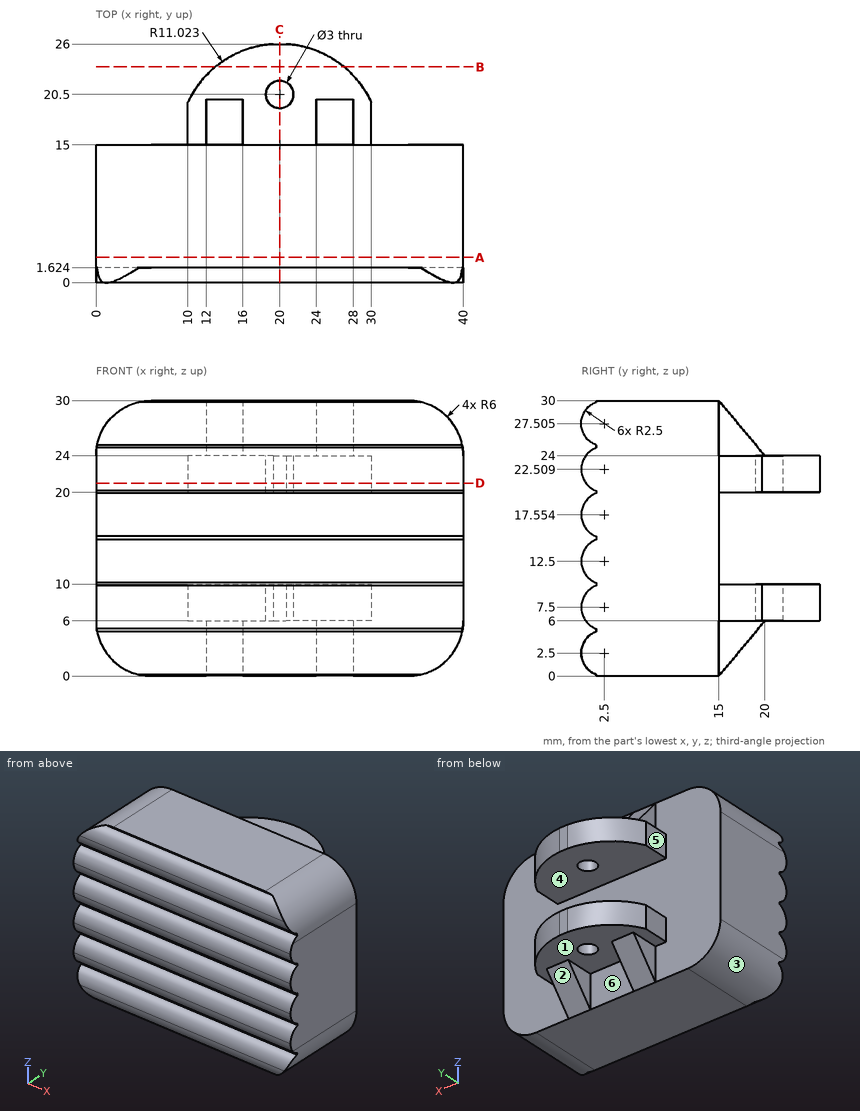
Geometry: see drawing. Coordinates: mm, zero at the bounding-box minimum. A direction names the side the tool comes from. Give positions to 0.01 mm unless a question says otherwise; leave off trailing zeros. Loops run counter-clockwise (first coordinate to the right, second up) from the corner with the lowest first, then second, coordinate; pieces in that order, holes last. Notation, with made-up numbers: (65, 87.25) - (98, 87.25) arc R13 ccw to (98, 94.25) - close; hole circle Ø11 at (-23.5, 16). An arc over 180 degrees is marked (long way). Use CSV: the item, a comma, the result in double quotes.
1) Pin query (flat end, axial travel): P1, Ø1, axis at y = 8.5, z = 27, coming from the +X side (1 decimal); P2, Ø8, axis at y = 22, z = 19, coming from the -X side; P3, Ø4, axis at y = 16.5, z = 1.5, coming from the +X side. Return the tip coordinate at first contact, or that it passes through.
Worked out:
P1,"stops at x = 39.5"
P2,"stops at x = 10"
P3,"stops at x = 39.09"
2) Line query: line 1 (Y direction, x = 20, z = 8); line 2 (Z direction, x = 23.5, y = 21.75); line 3 (X direction, y = 16.75, z = 8.5). Output: solid intervals per line, ascending.
Worked out:
line 1,"y = 0.05 to 19, 22 to 26"
line 2,"z = 6 to 10, 20 to 24"
line 3,"x = 10 to 30"
3) Cut plane C-C (x = 20). Count the separate pieces of the cut face and the enclosed holes in it.
Worked out:
separate pieces,"3"
enclosed holes,"0"
4) Cut plane A-A (y = 2.75). Output: boundary loops of the cut face in (x, z), and give its area (3 significant figures).
Worked out:
outline,"(0, 6) arc R6 ccw to (6, 0) - (34, 0) arc R6 ccw to (40, 6) - (40, 24) arc R6 ccw to (34, 30) - (6, 30) arc R6 ccw to (0, 24) - close"
area,"1,170 mm^2"
5) Cut plane B-B (y = 23.5). Output: boundary loops of the cut face in (x, z), and give its area (3 significant figures).
Worked out:
outline,"(12.98, 6) - (27.02, 6) - (27.02, 10) - (12.98, 10) - close; (12.98, 20) - (27.02, 20) - (27.02, 24) - (12.98, 24) - close"
area,"112 mm^2"
6) Set-up query: the marked faces 4, 5 and 6. Return all of +Z, -Z, +X, -X, +Y, -Y with unobstructed straight access to the full face (end or side cutting, diameter ignored); none if empty.
Worked out:
face 4,"+X, -X, +Y"
face 5,"+Z, -Z, -X, +Y"
face 6,"-Z, +Y"
7) Cut plane D-D (z = 21). Output: boundary loops of the cut face in (x, y) (1 decimal), and give its area (3 significant figures).
Worked out:
outline,"(0, 0.5) - (40, 0.5) - (40, 15) - (30, 15) - (30, 19.6) arc R11 ccw to (20.7, 26) - (19.3, 26) arc R11 ccw to (10, 19.6) - (10, 15) - (0, 15) - close; hole circle Ø3 at (20, 20.5)"
area,"757 mm^2"
8) Mould query, pull axis X, two halves, no side actions, for the marked faces 1, 2 and 3. Classes: +X half, -X half, draft (parallel to the pull), parting line (faces both ways), or undercut.
Worked out:
face 1,"undercut"
face 2,"draft"
face 3,"-X half"
